Source: CAD feature listing. Evaluate the final solid. Frame: model axes, mm. Face numbers are marked on the shaded views. Give positions to 0.01 mm unless a question says otherwise; leave off trailing zeros. Order: outer loops, then holes, each group sorted by start corner. A loop starts at its lowest first (then second) coordinate and runs counter-clockwise, first axis right, second up. Notation, with made-up numbers: M -3,-10.75 L 35,-10.75 A25 cw 35,10.25 Z; hole C 71,-33 d11. An arc over 180 degrees is marked long. Answer as a JSON object with one key per item and string values. Group by question number.
1. Section query A-A (z = 269.5). Output: boundary loops of the cut face in (x, y), plus the area to 3 significant figures.
2. Section query C-C (x = -25). Output: boundary loops of the cut face in (y, z).
3. Pin query (flat end, axial travel): P1, Ø5.5, axis at x = 1436.5, y = -12, coming from the +Z side; P2, Ø5.5, axis at y = -5, z = 369.5, coming from the -X side; P3, Ø4, axis at y = -5.5, z = 270, coming from the -X side; P4, Ø5, axis at x = 1080.5, z = 320.5, coming from the +Y side. Return the tip coordinate at first contact, or that it passes through.
4. Material intervals for L1, parallel to X at y = -3.75, z = 257; L2, parallel to X at y = -13.25, z = 293.5; L3, parallel to X at y = -14.25, z = 365.5, sorted ascending. Write a range as [from, to].
5. Pull-direction query (Y, two-part tool) for the marked faces 1 and 2; classes: +Y half, -Y half, draft (parallel to the pull), parting line (faces both ways), or undercut.
6. Section query B-B (x = 1328). Output: boundary loops of the cut face in (y, z).
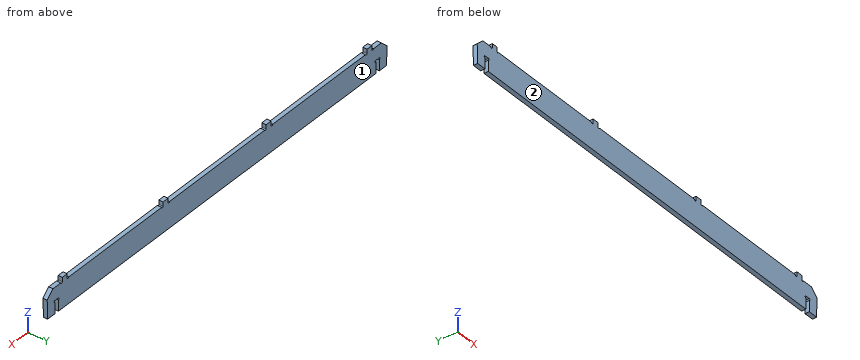
from build123d import *

# Parameters (mm, degrees)
F1_DEPTH = 18


# Not quite as in the source:
# - ends of sketch curves that miss each other by under 0.0002 mm in the source are joined


with BuildPart() as f1:
    # F0 (on Front) → F1 (new body)
    with BuildSketch(Plane.XZ):
        with BuildLine():
            Line((1444.9999982887, 361), (1444.9999982887, 379))
            Line((1444.9999982887, 379), (1418.9999982887, 379))
            Line((1418.9999982887, 379), (1418.9999982887, 361.0032042947))
            Line((1418.9999982887, 361.0032042947), (1418.9999982887, 361))
            ThreePointArc((1418.9999982887, 361), (1414.9978620926, 357.0032048651), (1410.9999984313, 361.0042723931))
            Line((1410.9999984313, 361.0042723931), (918.9999984313, 361.0042723931))
            ThreePointArc((918.9999984313, 361.0042723931), (914.9999984313, 357.0042723931), (910.9999984313, 361.0042723931))
            Line((910.9999984313, 361.0042723931), (910.9999984313, 379.0042723931))
            Line((910.9999984313, 379.0042723931), (884.9999984313, 379.0042723931))
            Line((884.9999984313, 379.0042723931), (884.9999984313, 361.0055952483))
            Line((884.9999984313, 361.0055952483), (884.9999984313, 361.0042723931))
            ThreePointArc((884.9999984313, 361.0042723931), (880.9986755762, 357.005595467), (876.9999986501, 361.0069181034))
            Line((876.9999986501, 361.0069181034), (372.9999978512, 361.1735978616))
            ThreePointArc((372.9999978512, 361.1735978616), (368.9986752099, 357.1749209454), (364.9999982887, 361.1762435819))
            Line((364.9999982887, 361.1762435819), (364.9999982887, 379.1762435819))
            Line((364.9999982887, 379.1762435819), (338.9999982887, 379.1762435819))
            Line((338.9999982887, 379.1762435819), (338.9999982887, 361.1783797782))
            ThreePointArc((338.9999982887, 361.1783797782), (334.9999982887, 357.1783797782), (330.9999982887, 361.1783797782))
            Line((330.9999982887, 361.1783797782), (-161.0000017113, 361.1783797782))
            ThreePointArc((-161.0000017113, 361.1783797782), (-165.0000017113, 357.1783797782), (-169.0000017113, 361.1783797782))
            Line((-169.0000017113, 361.1783797782), (-169.0000017113, 379.1783797782))
            Line((-169.0000017113, 379.1783797782), (-195.0000017113, 379.1783797782))
            Line((-195.0000017113, 379.1783797782), (-195.0000012844, 361.180516095))
            ThreePointArc((-195.0000012844, 361.180516095), (-198.9999999526, 357.1805172846), (-202.9999987156, 361.1805160001))
            Line((-202.9999987156, 361.1805160001), (-215.9862284595, 361.1805160001))
            Line((-215.9862284595, 361.1805160001), (-233.9862284595, 361.1805160001))
            Line((-233.9862284595, 361.1805160001), (-244.90749278, 361.1805160001))
            Line((-244.90749278, 361.1805160001), (-274.9862284595, 331.0746893941))
            Line((-274.9862284595, 331.0746893941), (-272.7034209311, 250.3365797868))
            Line((-272.7034209311, 250.3365797868), (-233.9862284595, 250.3365797868))
            Line((-233.9862284595, 250.3365797868), (-233.9862284595, 297.3365797868))
            ThreePointArc((-233.9862284595, 297.3365797868), (-237.9862284595, 301.3365797868), (-233.9862284595, 305.3365797868))
            Line((-233.9862284595, 305.3365797868), (-215.9862284595, 305.3365797868))
            ThreePointArc((-215.9862284595, 305.3365797868), (-211.9862284595, 301.3365797868), (-215.9862284595, 297.3365797868))
            Line((-215.9862284595, 297.3365797868), (-215.9862284595, 250.3365797868))
            Line((-215.9862284595, 250.3365797868), (-134.9862284595, 250.3365797868))
            Line((-134.9862284595, 250.3365797868), (1385.0137715405, 250.3365797868))
            Line((1385.0137715405, 250.3365797868), (1466.020051896, 250.3365797868))
            Line((1466.020051896, 250.3365797868), (1466.020051896, 297.3365797868))
            ThreePointArc((1466.020051896, 297.3365797868), (1462.020051896, 301.3365797868), (1466.020051896, 305.3365797868))
            Line((1466.020051896, 305.3365797868), (1484.020051896, 305.3365797868))
            ThreePointArc((1484.020051896, 305.3365797868), (1488.020051896, 301.3365797868), (1484.020051896, 297.3365797868))
            Line((1484.020051896, 297.3365797868), (1484.020051896, 250.3365797868))
            Line((1484.020051896, 250.3365797868), (1522.7328349544, 250.3365797868))
            Line((1522.7328349544, 250.3365797868), (1525.0137715405, 331))
            Line((1525.0137715405, 331), (1494.9069982887, 361))
            Line((1494.9069982887, 361), (1466.022162316, 361))
            Line((1466.022162316, 361), (1452.9999982887, 361))
            ThreePointArc((1452.9999982887, 361), (1448.9999982887, 357), (1444.9999982887, 361))
        make_face()
    extrude(amount=F1_DEPTH)


solid = f1.part
Answer sheet:
{
 "1": {"outline": "M -273.25,-18 L -233.99,-18 L -233.99,0 L -273.25,0 Z; M -215.99,-18 L 1466.02,-18 L 1466.02,0 L -215.99,0 Z; M 1484.02,-18 L 1523.27,-18 L 1523.27,0 L 1484.02,0 Z", "area": "31,700 mm^2"},
 "2": {"outline": "M -18,250.34 L 0,250.34 L 0,361.18 L -18,361.18 Z"},
 "3": {"P1": "z = 379", "P2": "x = -195", "P3": "x = -273.32", "P4": "y = 0"},
 "4": {"L1": "[-272.89, -233.99], [-215.99, 1466.02], [1484.02, 1522.92]", "L2": "[-273.92, -233.99], [-215.99, 1466.02], [1484.02, 1523.95]", "L3": "[-195, -169], [339, 365], [885, 911], [1419, 1445]"},
 "5": {"face 1": "+Y half", "face 2": "-Y half"},
 "6": {"outline": "M -18,250.34 L 0,250.34 L 0,361 L -18,361 Z"}
}
